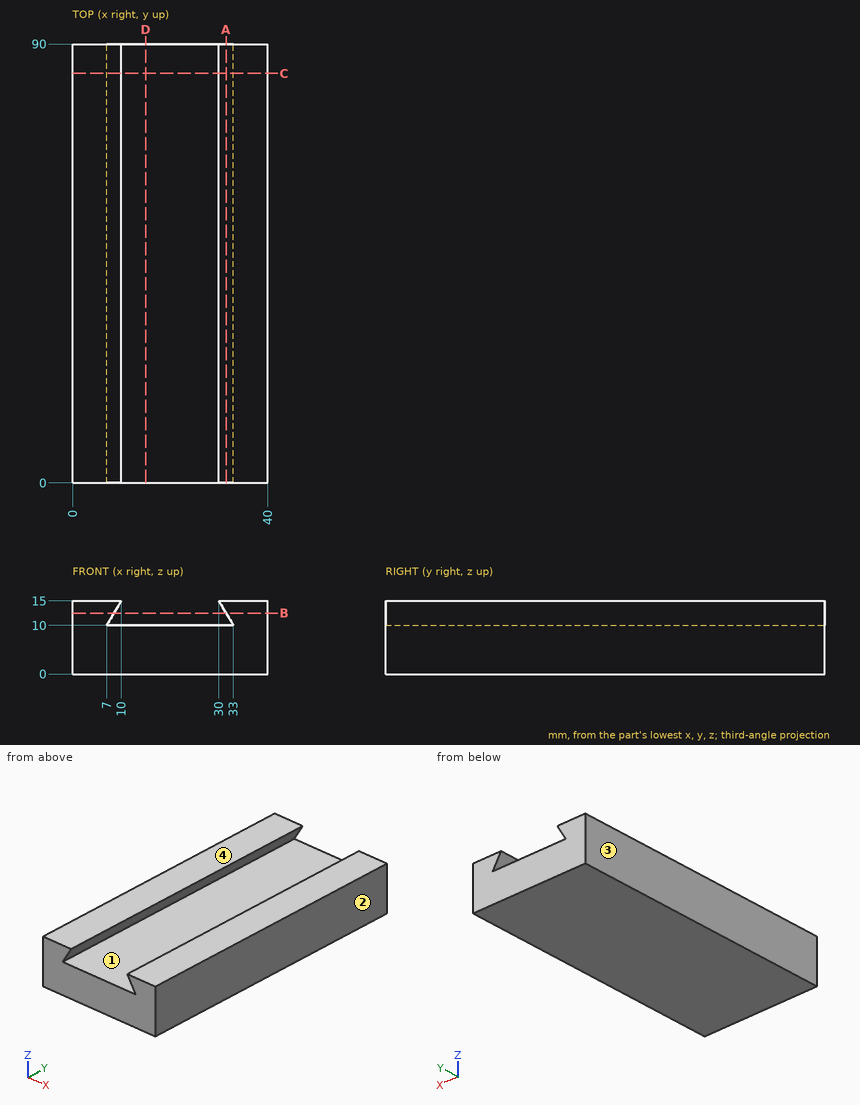
Answer from the drawing. Dimensions are ordinates in mm from the lowest x, y and z of the part. Give positions to 0.01 mm unless a question says otherwise; leave off trailing zeros. Loops run counter-clockwise (first coordinate to the right, second up) from the corner with the lowest first, then second, coordinate; pieces in that order, holes last. Notation, with made-up numbers: (38.5, -29) -> (79.5, -29) arc R26 ccw to (79.5, 0) -> close; hole circle Ø6 at (23.25, 47). An arc over 180 degrees is marked (long way). Use a Markdown table: item, result.
Q1. Determine the mould class of the marked faces 1, 2, 3 and 4 for opening direction X: pulls with the +X half, pulls with the -X half, needs draft (parallel to the pull), parting line crosses it, or undercut.
Solved:
| item | result |
|---|---|
| face 1 | undercut |
| face 2 | pulls with the +X half |
| face 3 | pulls with the -X half |
| face 4 | needs draft |
Q2. Section C-C, the plane y = 84 is taken. Determine the outline of the cut face in (x, z).
Solved:
| item | result |
|---|---|
| outline | (0, 0) -> (40, 0) -> (40, 15) -> (30, 15) -> (33, 10) -> (7, 10) -> (10, 15) -> (0, 15) -> close |
Q3. Find the intervals of material crossed by line 1 along Z through (x, y) = (27.5, 15.5); line 2 along Z through (x, y) = (8.5, 13); line 3 along X through (y, z) = (76, 11.75), in increasing order.
Solved:
| item | result |
|---|---|
| line 1 | z = 0 to 10 |
| line 2 | z = 0 to 10, 12.5 to 15 |
| line 3 | x = 0 to 8.05, 31.95 to 40 |
Q4. Section A-A, the plane x = 31.5 is taken. Determine the outline of the cut face in (y, z).
Solved:
| item | result |
|---|---|
| outline | (0, 0) -> (90, 0) -> (90, 10) -> (0, 10) -> close; (0, 12.5) -> (90, 12.5) -> (90, 15) -> (0, 15) -> close |
Q5. Section B-B, the plane z = 12.5 is taken. Determine the outline of the cut face in (x, y), then the cut area to 3 significant figures.
Solved:
| item | result |
|---|---|
| outline | (0, 0) -> (8.5, 0) -> (8.5, 90) -> (0, 90) -> close; (31.5, 0) -> (40, 0) -> (40, 90) -> (31.5, 90) -> close |
| area | 1,530 mm^2 |
Q6. Section D-D, the plane x = 15 is taken. Determine the outline of the cut face in (y, z), then the cut area to 3 significant figures.
Solved:
| item | result |
|---|---|
| outline | (0, 0) -> (90, 0) -> (90, 10) -> (0, 10) -> close |
| area | 900 mm^2 |
Q7. Each of these flat-tipped pins is pushed along its axis until it touches: pin 1 (21 mm diameter, centred on x = 26, y = 43, fed in from +Z); pin 2 (3 mm diameter, centred on x = 13.5, y = 35.5, fed in from +Z). Where does it stop, or does it pass through?
Solved:
| item | result |
|---|---|
| pin 1 | stops at z = 15 |
| pin 2 | stops at z = 10 |
